```python
from build123d import *

# Parameters (mm, degrees)
BOSS_EXTRUDE1_DEPTH      = 100
BOSS_EXTRUDE1_DEPTH_BACK = 65
CUT_EXTRUDE1_DEPTH       = 280


with BuildPart() as part:
    # Sketch1 → Boss-Extrude1 (new body, two sides)
    with BuildSketch(Plane.XY) as boss_extrude1_sk:
        Polygon((-140, 95), (-140, -95), (140, -95), (140, 95), (80, 235), (-80, 235), align=None)
    extrude(amount=BOSS_EXTRUDE1_DEPTH)
    extrude(boss_extrude1_sk.sketch, amount=-BOSS_EXTRUDE1_DEPTH_BACK)

    # Sketch2 → Cut-Extrude1 (cut)
    with BuildSketch(Plane(origin=(140, 0, 0), x_dir=(0, 0, -1), z_dir=(1, 0, 0))):
        with BuildLine():
            Line((-100, 190.377151129), (-100, 104.513728645))
            add(Edge.make_bspline(
                [(-100, 104.513728645), (-102.224477009, 93.061564682), (-100.352557358, 82.398786726), (-94.384241048, 72.525394779)],
                knots=[0, 0, 0, 0, 1, 1, 1, 1], degree=3))
            Line((-94.384241048, 72.525394779), (-86.862061889, 60.08144589))
            Line((-86.862061889, 60.08144589), (-86.862061889, -67.213116322))
            add(Edge.make_bspline(
                [(-86.862061889, -67.213116322), (-95.040230762, -73.563203777), (-104.810422505, -83.101213531), (-100, -95)],
                knots=[0, 0, 0, 0, 1, 1, 1, 1], degree=3))
            Line((-100, -95), (-158.360908781, -95))
            Line((-158.360908781, -95), (-158.360908781, 235))
            Line((-158.360908781, 235), (-71.936287457, 235))
            add(Edge.make_bspline(
                [(-71.936287457, 235), (-104.052371602, 224.516044217), (-100, 190.377151129)],
                knots=[0, 0, 0, 1, 1, 1], degree=2))
        make_face()
    extrude(amount=-CUT_EXTRUDE1_DEPTH, mode=Mode.SUBTRACT)


solid = part.part
```
Check sheet for the modelled part. Datum: model origin and axes. Units: mm. A direction names the side the tool comes from. Give positions to 0.01 mm unless a question says otherwise; leave off trailing zeros. Order: outer loops, then holes, each group sorted by start corner. A loop starts at its lowest first (then second) coordinate and runs counter-clockwise, first axis right, second up. Notation, with made-up numbers: M 30.5,-23.75 L 38.5,-23.75 A24 ccw 38.5,8.25 Z; hole C -35.75,-24.75 d11. An arc over 180 degrees is marked long. Answer in a Markdown table with one row per item. Add a question column.
Q1. Release check for a two-part mould opening along Y. For faces 3 (the flat face through (-140, 1, 19)), 4 (the flat face through (-109.58, 165.98, 18.66)), 5 (the flat face through (2, -3, 86.862)) record: released by +Y, released by -Y, zero draft, split by the parting line, or undercut.
Q2. Thickness scan on L1, parallel to Z at x = -12, y = 21.5; L2, parallel to Y at x = 86.5, z = 84; L3, parallel to Y at x = 88, z = 67. Record the ranges inside material, lowest first.
Q3. Gauge pin test, flat end, axial feed: pin 1 Ø6 at (x, z) = (87.5, -22) entering from +Y. Record the tip position at first contact, or that the pin passes through.
Q4. Access from +Z, -Z, +X, -X, +Y, -Y to the whole of each face (thin tool, end or side, straight path). Record for faces 1 (the flat face through (1.96, 66.391, 90.676)), 2 (the flat face through (-2, 146, 100)).
Q5. Sectioned sample at A-A, the plane z = -46. Record the boundary of the cut face in (x, y).
Q6. Sectioned sample at C-C, the plane y = 121. Record the boundary of the cut face in (x, z), and give its area (3 significant figures).
Q7. Sectioned sample at B-B, the plane y = 41. Record the boundary of the cut face in (x, z).
Verdict:
| question | item | result |
|---|---|---|
| 1 | face 3 | zero draft |
| 1 | face 4 | released by +Y |
| 1 | face 5 | undercut |
| 2 | L1 | -65 to 86.86 |
| 2 | L2 | -95 to 219.83 |
| 2 | L3 | -95 to 216.33 |
| 3 | pin 1 | y = 224.5 |
| 4 | face 1 | +Z, +X, -X |
| 4 | face 2 | +Z, +X, -X, +Y, -Y |
| 5 | outline | M -140,-95 L 140,-95 L 140,95 L 80,235 L -80,235 L -140,95 Z |
| 6 | outline | M -128.86,-65 L 128.86,-65 L 128.86,100 L -128.86,100 Z |
| 6 | area | 42,500 mm² |
| 7 | outline | M -140,-65 L 140,-65 L 140,86.86 L -140,86.86 Z |
